from build123d import *

# Parameters (mm, degrees)
SKETCH1_W                      = 132
SKETCH1_H                      = 80
BOSS_EXTRUDE1_DEPTH            = 5
SKETCH3_R                      = 3.5
SKETCH3_R_2                    = 2.5
BOSS_EXTRUDE2_DEPTH            = 9
CUT_EXTRUDE1_REACH             = 7
SKETCH2_R                      = 1.6
CUT_EXTRUDE1_DIRECTION_2_REACH = 11
SKETCH4_R                      = 3.05
CUT_EXTRUDE2_DEPTH             = 3.2
CUT_EXTRUDE3_REACH             = 7
SKETCH5_R                      = 1.6
CUT_EXTRUDE4_DEPTH             = 1.5


with BuildPart() as part:
    # Sketch1 → Boss-Extrude1 (new body)
    with BuildSketch(Plane(origin=(0, 0, 0), x_dir=(1, 0, 0), z_dir=(0, 1, 0))):
        Rectangle(SKETCH1_W, SKETCH1_H)
    extrude(amount=BOSS_EXTRUDE1_DEPTH)

    # Sketch3 → Boss-Extrude2 (add)
    with BuildSketch(Plane(origin=(0, 5, 0), x_dir=(1, 0, 0), z_dir=(0, 1, 0))):
        with Locations((-58.921474433, 28.5)):
            Circle(SKETCH3_R)
        with Locations((15.578525567, 28.5)):
            Circle(SKETCH3_R)
        with Locations((15.578525567, -28.5)):
            Circle(SKETCH3_R)
        with Locations((-58.921474433, -28.5)):
            Circle(SKETCH3_R)
        with Locations((25.378681006, -28.5)):
            Circle(SKETCH3_R_2)
        with Locations((59.178681006, -28.5)):
            Circle(SKETCH3_R_2)
        with Locations((42.278681006, 8)):
            Circle(SKETCH3_R_2)
    extrude(amount=BOSS_EXTRUDE2_DEPTH)

    # Sketch2 → Cut-Extrude1 (cut, up to next)
    with BuildSketch(Plane(origin=(0, 5, 0), x_dir=(1, 0, 0), z_dir=(0, 1, 0)), mode=Mode.PRIVATE) as cut_extrude1_sk1:
        with Locations((42.278681006, 8)):
            Circle(SKETCH2_R)
    cut_extrude1_tool1 = extrude(cut_extrude1_sk1.sketch, amount=-CUT_EXTRUDE1_REACH, mode=Mode.PRIVATE) & part.part
    add(cut_extrude1_tool1.solids().sort_by_distance((42.278681, 5, -8))[0], mode=Mode.SUBTRACT)
    # Sketch2 → Cut-Extrude1 (cut, up to next)
    with BuildSketch(Plane(origin=(0, 5, 0), x_dir=(1, 0, 0), z_dir=(0, 1, 0)), mode=Mode.PRIVATE) as cut_extrude1_sk2:
        with Locations((25.378681006, -28.5)):
            Circle(SKETCH2_R)
    cut_extrude1_tool2 = extrude(cut_extrude1_sk2.sketch, amount=-CUT_EXTRUDE1_REACH, mode=Mode.PRIVATE) & part.part
    add(cut_extrude1_tool2.solids().sort_by_distance((25.378681, 5, 28.5))[0], mode=Mode.SUBTRACT)
    # Sketch2 → Cut-Extrude1 (cut, up to next)
    with BuildSketch(Plane(origin=(0, 5, 0), x_dir=(1, 0, 0), z_dir=(0, 1, 0)), mode=Mode.PRIVATE) as cut_extrude1_sk3:
        with Locations((59.178681006, -28.5)):
            Circle(SKETCH2_R)
    cut_extrude1_tool3 = extrude(cut_extrude1_sk3.sketch, amount=-CUT_EXTRUDE1_REACH, mode=Mode.PRIVATE) & part.part
    add(cut_extrude1_tool3.solids().sort_by_distance((59.178681, 5, 28.5))[0], mode=Mode.SUBTRACT)
    # Sketch2 → Cut-Extrude1 (cut, up to next)
    with BuildSketch(Plane(origin=(0, 5, 0), x_dir=(1, 0, 0), z_dir=(0, 1, 0)), mode=Mode.PRIVATE) as cut_extrude1_sk4:
        with Locations((15.578525567, 28.5)):
            Circle(SKETCH2_R)
    cut_extrude1_tool4 = extrude(cut_extrude1_sk4.sketch, amount=-CUT_EXTRUDE1_REACH, mode=Mode.PRIVATE) & part.part
    add(cut_extrude1_tool4.solids().sort_by_distance((15.578526, 5, -28.5))[0], mode=Mode.SUBTRACT)
    # Sketch2 → Cut-Extrude1 (cut, up to next)
    with BuildSketch(Plane(origin=(0, 5, 0), x_dir=(1, 0, 0), z_dir=(0, 1, 0)), mode=Mode.PRIVATE) as cut_extrude1_sk5:
        with Locations((15.578525567, -28.5)):
            Circle(SKETCH2_R)
    cut_extrude1_tool5 = extrude(cut_extrude1_sk5.sketch, amount=-CUT_EXTRUDE1_REACH, mode=Mode.PRIVATE) & part.part
    add(cut_extrude1_tool5.solids().sort_by_distance((15.578526, 5, 28.5))[0], mode=Mode.SUBTRACT)
    # Sketch2 → Cut-Extrude1 (cut, up to next)
    with BuildSketch(Plane(origin=(0, 5, 0), x_dir=(1, 0, 0), z_dir=(0, 1, 0)), mode=Mode.PRIVATE) as cut_extrude1_sk6:
        with Locations((-58.921474433, -28.5)):
            Circle(SKETCH2_R)
    cut_extrude1_tool6 = extrude(cut_extrude1_sk6.sketch, amount=-CUT_EXTRUDE1_REACH, mode=Mode.PRIVATE) & part.part
    add(cut_extrude1_tool6.solids().sort_by_distance((-58.921474, 5, 28.5))[0], mode=Mode.SUBTRACT)
    # Sketch2 → Cut-Extrude1 (cut, up to next)
    with BuildSketch(Plane(origin=(0, 5, 0), x_dir=(1, 0, 0), z_dir=(0, 1, 0)), mode=Mode.PRIVATE) as cut_extrude1_sk7:
        with Locations((-58.921474433, 28.5)):
            Circle(SKETCH2_R)
    cut_extrude1_tool7 = extrude(cut_extrude1_sk7.sketch, amount=-CUT_EXTRUDE1_REACH, mode=Mode.PRIVATE) & part.part
    add(cut_extrude1_tool7.solids().sort_by_distance((-58.921474, 5, -28.5))[0], mode=Mode.SUBTRACT)

    # Sketch2 → Cut-Extrude1 direction 2 (cut, up to next)
    with BuildSketch(Plane(origin=(0, 5, 0), x_dir=(1, 0, 0), z_dir=(0, 1, 0)), mode=Mode.PRIVATE) as cut_extrude1_direction_2_sk1:
        with Locations((42.278681006, 8)):
            Circle(SKETCH2_R)
    cut_extrude1_direction_2_tool1 = extrude(cut_extrude1_direction_2_sk1.sketch, amount=CUT_EXTRUDE1_DIRECTION_2_REACH, mode=Mode.PRIVATE) & part.part
    add(cut_extrude1_direction_2_tool1.solids().sort_by_distance((42.278681, 5, -8))[0], mode=Mode.SUBTRACT)
    # Sketch2 → Cut-Extrude1 direction 2 (cut, up to next)
    with BuildSketch(Plane(origin=(0, 5, 0), x_dir=(1, 0, 0), z_dir=(0, 1, 0)), mode=Mode.PRIVATE) as cut_extrude1_direction_2_sk2:
        with Locations((25.378681006, -28.5)):
            Circle(SKETCH2_R)
    cut_extrude1_direction_2_tool2 = extrude(cut_extrude1_direction_2_sk2.sketch, amount=CUT_EXTRUDE1_DIRECTION_2_REACH, mode=Mode.PRIVATE) & part.part
    add(cut_extrude1_direction_2_tool2.solids().sort_by_distance((25.378681, 5, 28.5))[0], mode=Mode.SUBTRACT)
    # Sketch2 → Cut-Extrude1 direction 2 (cut, up to next)
    with BuildSketch(Plane(origin=(0, 5, 0), x_dir=(1, 0, 0), z_dir=(0, 1, 0)), mode=Mode.PRIVATE) as cut_extrude1_direction_2_sk3:
        with Locations((59.178681006, -28.5)):
            Circle(SKETCH2_R)
    cut_extrude1_direction_2_tool3 = extrude(cut_extrude1_direction_2_sk3.sketch, amount=CUT_EXTRUDE1_DIRECTION_2_REACH, mode=Mode.PRIVATE) & part.part
    add(cut_extrude1_direction_2_tool3.solids().sort_by_distance((59.178681, 5, 28.5))[0], mode=Mode.SUBTRACT)
    # Sketch2 → Cut-Extrude1 direction 2 (cut, up to next)
    with BuildSketch(Plane(origin=(0, 5, 0), x_dir=(1, 0, 0), z_dir=(0, 1, 0)), mode=Mode.PRIVATE) as cut_extrude1_direction_2_sk4:
        with Locations((15.578525567, 28.5)):
            Circle(SKETCH2_R)
    cut_extrude1_direction_2_tool4 = extrude(cut_extrude1_direction_2_sk4.sketch, amount=CUT_EXTRUDE1_DIRECTION_2_REACH, mode=Mode.PRIVATE) & part.part
    add(cut_extrude1_direction_2_tool4.solids().sort_by_distance((15.578526, 5, -28.5))[0], mode=Mode.SUBTRACT)
    # Sketch2 → Cut-Extrude1 direction 2 (cut, up to next)
    with BuildSketch(Plane(origin=(0, 5, 0), x_dir=(1, 0, 0), z_dir=(0, 1, 0)), mode=Mode.PRIVATE) as cut_extrude1_direction_2_sk5:
        with Locations((15.578525567, -28.5)):
            Circle(SKETCH2_R)
    cut_extrude1_direction_2_tool5 = extrude(cut_extrude1_direction_2_sk5.sketch, amount=CUT_EXTRUDE1_DIRECTION_2_REACH, mode=Mode.PRIVATE) & part.part
    add(cut_extrude1_direction_2_tool5.solids().sort_by_distance((15.578526, 5, 28.5))[0], mode=Mode.SUBTRACT)
    # Sketch2 → Cut-Extrude1 direction 2 (cut, up to next)
    with BuildSketch(Plane(origin=(0, 5, 0), x_dir=(1, 0, 0), z_dir=(0, 1, 0)), mode=Mode.PRIVATE) as cut_extrude1_direction_2_sk6:
        with Locations((-58.921474433, -28.5)):
            Circle(SKETCH2_R)
    cut_extrude1_direction_2_tool6 = extrude(cut_extrude1_direction_2_sk6.sketch, amount=CUT_EXTRUDE1_DIRECTION_2_REACH, mode=Mode.PRIVATE) & part.part
    add(cut_extrude1_direction_2_tool6.solids().sort_by_distance((-58.921474, 5, 28.5))[0], mode=Mode.SUBTRACT)
    # Sketch2 → Cut-Extrude1 direction 2 (cut, up to next)
    with BuildSketch(Plane(origin=(0, 5, 0), x_dir=(1, 0, 0), z_dir=(0, 1, 0)), mode=Mode.PRIVATE) as cut_extrude1_direction_2_sk7:
        with Locations((-58.921474433, 28.5)):
            Circle(SKETCH2_R)
    cut_extrude1_direction_2_tool7 = extrude(cut_extrude1_direction_2_sk7.sketch, amount=CUT_EXTRUDE1_DIRECTION_2_REACH, mode=Mode.PRIVATE) & part.part
    add(cut_extrude1_direction_2_tool7.solids().sort_by_distance((-58.921474, 5, -28.5))[0], mode=Mode.SUBTRACT)

    # Sketch4 → Cut-Extrude2 (cut)
    with BuildSketch(Plane.XZ):
        with Locations((42.278681006, -8)):
            Circle(SKETCH4_R)
        with Locations((59.178681006, 28.5)):
            Circle(SKETCH4_R)
        with Locations((25.378681006, 28.5)):
            Circle(SKETCH4_R)
        with Locations((15.578525567, 28.5)):
            Circle(SKETCH4_R)
        with Locations((15.578525567, -28.5)):
            Circle(SKETCH4_R)
        with Locations((-58.921474433, -28.5)):
            Circle(SKETCH4_R)
        with Locations((-58.921474433, 28.5)):
            Circle(SKETCH4_R)
    extrude(amount=-CUT_EXTRUDE2_DEPTH, mode=Mode.SUBTRACT)

    # Sketch5 → Cut-Extrude3 (cut, up to next)
    with BuildSketch(Plane(origin=(0, 5, 0), x_dir=(1, 0, 0), z_dir=(0, 1, 0)), mode=Mode.PRIVATE) as cut_extrude3_sk1:
        with Locations((-35.011855655, -13.657285002)):
            Circle(SKETCH5_R)
    cut_extrude3_tool1 = extrude(cut_extrude3_sk1.sketch, amount=-CUT_EXTRUDE3_REACH, mode=Mode.PRIVATE) & part.part
    add(cut_extrude3_tool1.solids().sort_by_distance((-35.011856, 5, 13.657285))[0], mode=Mode.SUBTRACT)
    # Sketch5 → Cut-Extrude3 (cut, up to next)
    with BuildSketch(Plane(origin=(0, 5, 0), x_dir=(1, 0, 0), z_dir=(0, 1, 0)), mode=Mode.PRIVATE) as cut_extrude3_sk2:
        with Locations((41.861471436, 29.814909243)):
            Circle(SKETCH5_R)
    cut_extrude3_tool2 = extrude(cut_extrude3_sk2.sketch, amount=-CUT_EXTRUDE3_REACH, mode=Mode.PRIVATE) & part.part
    add(cut_extrude3_tool2.solids().sort_by_distance((41.861471, 5, -29.814909))[0], mode=Mode.SUBTRACT)

    # Sketch6 → Cut-Extrude4 (cut)
    with BuildSketch(Plane(origin=(0, 5, 0), x_dir=(1, 0, 0), z_dir=(0, 1, 0))):
        Polygon((-33.395274901, -16.457285002), (-31.778694147, -13.657285002), (-33.395274901, -10.857285002), (-36.628436408, -10.857285002), (-38.245017162, -13.657285002), (-36.628436408, -16.457285002), align=None)
        Polygon((43.478052189, 27.014909243), (45.094632943, 29.814909243), (43.478052189, 32.614909243), (40.244890682, 32.614909243), (38.628309928, 29.814909243), (40.244890682, 27.014909243), align=None)
    extrude(amount=-CUT_EXTRUDE4_DEPTH, mode=Mode.SUBTRACT)


solid = part.part
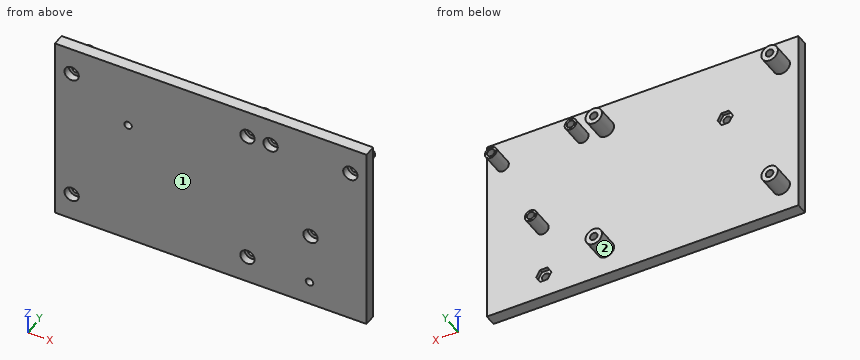
Design review of the part built by this model. Coordinates are the model's own, in mm. Face numbers are marked on the shaded views. Coordinates: 2 decimals unless noted, no trailing zeros. Order: outer loops, then holes, each group sorted by start corner. A loop starts at its lowest first (then second) coordinate and runs counter-clockwise, first axis right, second up. Notation, with made-up numbers: (-11.5, -33.5) -> (25.5, -33.5) arc R20 ccw to (25.5, -7.5) -> close; hole circle Ø10 at (23.25, -4). An arc over 180 degrees is marked (long way). Use one line per item in the form item = value. Start each with the question number.
(1) The part is to be moulded in two halves that separate along Z. For the marked faces 1 and 2, say which applies: +Z half, -Z half, draft (parallel to the pull), parting line (faces both ways), or undercut.
(2) Add section B-B on z = -8. State the section outline as (x, y) points, plus the area to 3 significant figures.
(3) Insertion check: pin 1 (8 mm diameter, centred on x = -24.5, z = -23, fed in from +Y); pin 2 (1.9 mm diameter, centred on x = 15.58, z = -28.5, fed in from -Y); pin 3 (1.8 mm diameter, centred on x = 26.5, z = 30, fed in from -Y); pin 4 (1.5 mm diameter, centred on x = 44, y = 10.5, fed in from -Z). Each pin has a flat end and moves straight along its axis. Give the tip position at first contact, or say it passes through.
(4) Add section D-D on x = 48. State the section outline as (y, z) points.
(5) Add section A-A on y = 11.75. Give the number of separate pieces and of enclosed holes in the cut face, plus the area to 3 significant figures.
(6) For probe 1 along Z at (x, y) = (-59, 7.75); probe 2 along Z at (x, y) = (25, 1.5); probe 3 along Z at (x, y) = (-59, 2.75), list the stretches that pass through material, from the lowest coordinate up.
Answer block:
q1.face_1 = draft
q1.face_2 = undercut
q2.outline = (-66, 0) -> (39.23, 0) -> (39.23, 3.2) -> (40.68, 3.2) -> (40.68, 14) -> (39.78, 14) -> (39.78, 5) -> (-66, 5) -> close; (43.88, 3.2) -> (45.33, 3.2) -> (45.33, 0) -> (66, 0) -> (66, 5) -> (44.78, 5) -> (44.78, 14) -> (43.88, 14) -> close
q2.area = 651 mm²
q3.pin_1 = 5
q3.pin_2 = through
q3.pin_3 = 3.2
q3.pin_4 = -10.3
q4.outline = (0, -40) -> (5, -40) -> (5, 40) -> (0, 40) -> close
q5.separate_pieces = 7
q5.enclosed_holes = 7
q5.area = 157 mm²
q6.probe_1 = -32 to -30.1, -26.9 to -25, 25 to 26.9, 30.1 to 32
q6.probe_2 = -40 to 25.47, 31.53 to 40
q6.probe_3 = -40 to -31.55, -25.45 to 25.45, 31.55 to 40
